from build123d import *

# Parameters (mm, degrees)
SKETCH1_R           = 20
SKETCH1_R_2         = 2.5
BOSS_EXTRUDE1_DEPTH = 2.5


with BuildPart() as part:
    # Sketch1 → Boss-Extrude1 (new body)
    with BuildSketch(Plane.XY):
        with BuildLine():
            Line((-80, 45), (80, 45))
            ThreePointArc((80, 45), (125, 0), (80, -45))
            Line((80, -45), (30, -125))
            ThreePointArc((30, -125), (0, -155), (-30, -125))
            Line((-30, -125), (-80, -45))
            ThreePointArc((-80, -45), (-125, 0), (-80, 45))
        make_face()
        with Locations((-80, 0)):
            Circle(SKETCH1_R, mode=Mode.SUBTRACT)
        with Locations((80, 0)):
            Circle(SKETCH1_R, mode=Mode.SUBTRACT)
        Circle(SKETCH1_R_2, mode=Mode.SUBTRACT)
        with Locations((0, -125)):
            Circle(SKETCH1_R_2, mode=Mode.SUBTRACT)
    extrude(amount=BOSS_EXTRUDE1_DEPTH)


solid = part.part
Geometry: final body of the model. Coordinates: model frame, mm. Coordinates: 2 decimals unless noted, no trailing zeros. Order: outer loops, then holes, each group sorted by start corner. A loop starts at its lowest first (then second) coordinate and runs counter-clockwise, first axis right, second up.
(1) Material intervals for probe 1 along Y at (x, z) = (-80, 0.5); probe 2 along X at (y, z) = (-16.5, 2.2); probe 3 along Y at (x, z) = (93, 0.4), sorted ascending.
(2) Draft query along Y for faces 1 (the face through (-0.54, -2.44, 1.23)), 2 (the face through (-124.99, -0.99, 1.23)), 3 (the face through (55.35, -84.44, 1.23)). Return one class per face: pulls with the +Y half, pulls with the -Y half, needs draft (parallel to the pull), parting line crosses it, or undercut.
(3) Section query B-B (x = -40.5). Return the cut outline in (y, z).
(4) Section query C-C (y = -26.5). Return the cut outline in (x, z).
(5) First-contact query: pin 1 (1 mm diameter, centred on x = -82, z = 1, fed in from +Y) (3 decimals). Flat tip, straight axial feed; report the tip coordinate or a pass-through.
(6) Section query A-A (z = 1.65). Return the cut outline in (x, y), plus the area to 3 significant figures.
Solution:
1. probe 1: y = -45 to -20, 20 to 45
1. probe 2: x = -121.87 to -91.3, -68.7 to 68.7, 91.3 to 121.87
1. probe 3: y = -43.08 to -15.2, 15.2 to 43.08
2. face 1: undercut
2. face 2: parting line crosses it
2. face 3: pulls with the -Y half
3. outline: (-108.2, 0) - (45, 0) - (45, 2.5) - (-108.2, 2.5) - close
4. outline: (-116.37, 0) - (116.37, 0) - (116.37, 2.5) - (-116.37, 2.5) - close
5. pin 1: stops at y = 44.975
6. outline: (-80, -45) - (-30, -125) arc R30 ccw to (30, -125) - (80, -45) arc R45 ccw to (80, 45) - (-80, 45) arc R45 ccw to start; hole circle Ø40 at (-80, 0); hole circle Ø5 at (0, -125); hole circle Ø5 at (0, 0); hole circle Ø40 at (80, 0)
6. area: 28,400 mm2
